```python
from build123d import *

# Parameters (mm, degrees)
SKETCH_3_W          = 24
SKETCH_3_H          = 24
EXTRUDE_1_DEPTH     = 20
CUT_EXTRUDE_1_REACH = 28.23
SKETCH_4_R          = 10
SKETCH_6_W          = 24
SKETCH_6_H          = 24
EXTRUDE_2_DEPTH     = 20
SKETCH_8_R          = 3.25
CUT_EXTRUDE_2_DEPTH = 54.677075735


with BuildPart() as part:
    # 草图3 → 凸台-拉伸1 (new body)
    with BuildSketch(Plane.XY.offset(26.489014396)):
        Rectangle(SKETCH_3_W, SKETCH_3_H)
    extrude(amount=-EXTRUDE_1_DEPTH)

    # 草图4 → 切除-拉伸1 (cut, up to next)
    with BuildSketch(Plane(origin=(0, 0, 6.489014396), x_dir=(-1, 0, 0), z_dir=(0, 0, -1)), mode=Mode.PRIVATE) as cut_extrude_1_sk1:
        Circle(SKETCH_4_R)
    cut_extrude_1_tool1 = extrude(cut_extrude_1_sk1.sketch, amount=-CUT_EXTRUDE_1_REACH, mode=Mode.PRIVATE) & part.part
    add(cut_extrude_1_tool1.solids().sort_by_distance((0, 0, 6.489014))[0], mode=Mode.SUBTRACT)

    # 草图6 → 凸台-拉伸2 (add)
    with BuildSketch(Plane.XY.offset(26.489014396)):
        Rectangle(SKETCH_6_W, SKETCH_6_H)
    extrude(amount=EXTRUDE_2_DEPTH)

    # 草图8 → 切除-拉伸2 (cut, through all)
    with BuildSketch(Plane(origin=(12, 0, 0), x_dir=(0, 0, -1), z_dir=(1, 0, 0))):
        with Locations(Location((-16.989014396, 0, 0), (0, 0, 90))):
            Circle(SKETCH_8_R)
    extrude(amount=-CUT_EXTRUDE_2_DEPTH, mode=Mode.SUBTRACT)


solid = part.part
```
Work out the finished part from the listing and answer in its coordinate system (mm). A direction names the side the tool comes from. Round coordinates to 2 decimals unless told otherwise and drop trailing zeros. Write each loop counter-clockwise with the first axis right and the second up, starting at its lowest first coordinate (ties: lowest second). Pieces come first, ordered by that corner, then holes.
1) Consider probe 1 along X at (y, z) = (0, 12); probe 2 along Z at (x, y) = (-10.1, 0). Determine where each line is inside the solid, lowest interval first.
2) Determine the mould class of faces 1 (the face through (0, 0, 26.489)), 2 (the face through (-12, 0, 26)), 3 (the face through (0, 0, 46.489)) for opening direction X: pulls with the +X half, pulls with the -X half, needs draft (parallel to the pull), parting line crosses it, or undercut.
3) A cutting plane is placed at D-D on z = 23.5. Determine the outline of the cut face in (x, y).
4) A cutting plane is placed at C-C on x = 0. Determine the outline of the cut face in (y, z), and give its area (3 significant figures).
5) A cutting plane is placed at A-A on y = 0. Determine the outline of the cut face in (x, z), and give its area (3 significant figures).
6) A cutting plane is placed at B-B on y = -8. Determine the outline of the cut face in (x, z).
7) Which of the six approach directions +Z, -Z, +X, -X, +Y, -Y give full straight-line access (tool end or side, diameter ignored) to faces 4 (the face through (-9.237, -3.83, 16.349)), 5 (the face through (10.75, 3.1, 17.97))?
8) A flat-ended cylindrical pin translates along its axis: P1, Ø12, axis at x = 0, y = 0, coming from the -Z side. Find the tip coordinate at first contact, or state that the pin passes through.
Entries:
1. probe 1: x = -12 to -10, 10 to 12
1. probe 2: z = 6.49 to 13.74, 20.24 to 46.49
2. face 1: undercut
2. face 2: pulls with the -X half
2. face 3: needs draft
3. outline: (-12, -12) - (12, -12) - (12, 12) - (-12, 12) - close; hole circle Ø20 at (0, 0)
4. outline: (-12, 6.49) - (-10, 6.49) - (-10, 26.49) - (10, 26.49) - (10, 6.49) - (12, 6.49) - (12, 46.49) - (-12, 46.49) - close
4. area: 560 mm2
5. outline: (-12, 6.49) - (-10, 6.49) - (-10, 13.74) - (-12, 13.74) - close; (-12, 20.24) - (-10, 20.24) - (-10, 26.49) - (10, 26.49) - (10, 20.24) - (12, 20.24) - (12, 46.49) - (-12, 46.49) - close; (10, 6.49) - (12, 6.49) - (12, 13.74) - (10, 13.74) - close
5. area: 534 mm2
6. outline: (-12, 6.49) - (-6, 6.49) - (-6, 26.49) - (6, 26.49) - (6, 6.49) - (12, 6.49) - (12, 46.49) - (-12, 46.49) - close
7. face 4: -Z
7. face 5: +X, -X
8. P1: stops at z = 26.49
